Autodesk Inventor part; units mm, degrees
ref_plane "YZ Plane" through (0, 0, 0) normal (1, 0, 0) x (0, 1, 0)
ref_plane "XZ Plane" through (0, 0, 0) normal (0, 1, 0) x (-1, 0, 0)
ref_plane "XY Plane" through (0, 0, 0) normal (0, 0, 1) x (1, 0, 0)
sketch "Sketch1" plane through (0, 0, 0) normal (0, 0, 1) x (1, 0, 0)
  line L0 (0, 0) -> (73.025, 0)
  line L1 (73.025, 0) -> (73.025, 25.4)
  line L2 (73.025, 25.4) -> (-25.4001, 76.2)
  line L3 (-25.4001, 76.2) -> (-45.7201, 60.9599)
  line L4 (-45.7201, 60.9599) -> (0, 0)
  circle A0 centre (60.325, 12.7) radius 3.3734
  circle A1 centre (34.925, 12.7) radius 3.3734
  circle A2 centre (2.54, 17.78) radius 3.3734
  circle A3 centre (-27.9401, 58.42) radius 3.3734
  line L5 (73.025, 12.7) -> (-9.525, 12.7) construction
  line L6 (-35.5601, 68.5799) -> (15.875, 0) construction
  line L7 (0, 0) -> (49.8292, 37.372) construction
  line L8 (20.32, 15.24) -> (12.7, 25.4) construction
  circle A4 centre (-12.7001, 38.1) radius 3.3734
  dimension "d0" = 73.025
  dimension "d1" = 25.4
  dimension "d2" = 25.4
  dimension "d3" = 76.2
  dimension "d4" = 126.87
  dimension "d5" = 6.7469
  dimension "d6" = 25.4
  dimension "d7" = 12.7
  dimension "d8" = 12.7
  dimension "d12" = 12.7
  dimension "d13" = 25.4
  dimension "d14" = 12.7
  dimension "d15" = 38.1
extrude "Extrusion1" add sketch "Sketch1" along normal blind 3.175 contours L4 L3 L2 L1 L0 | A4
properties part number "angle gusset plate"
Can you work these out from the model? Positions are in its coordinate system, mm. Give positions to 0.01 mm unless a question says otherwise; leave off trailing zeros. Order: outer loops, then holes, each group sorted by start corner. A loop starts at its lowest first (then second) coordinate and runs counter-clockwise, first axis right, second up. Notation, with made-up numbers: (83, -31) - (97, -31) arc R29 cw to (97, 2) - close; hole circle Ø2 at (57.25, 76). An arc over 180 degrees is marked (long way). Use a Markdown table: item, result. Add a question column.
Q1. Please list where these lines run through material, in increasing order: line 1 along X through (y, z) = (14, 2.5) (3 decimals); line 2 along Y through (x, z) = (2.54, 1.05); line 3 along Y through (x, z) = (36, 1.85).
Q2. If we section it at B-B on y = 17.78: Write out the boundary of the cut face in (x, z) (3 decimals), plus the area to 3 significant figures.
Q3. If we section it at A-A on z = 0.55: Write out the boundary of the cut face in (x, y) (3 decimals).
Q4. If we section it at D-D on y = 39.5: Write out the boundary of the cut face in (x, z) (3 decimals), plus the area to 3 significant figures.
Q5. I'm going to push flat-ended pins straight in: pin 1 (4 mm diameter, centred on x = -27.94, y = 58.42, fed in from +Z); pin 2 (11 mm diameter, centred on x = 60.325, y = 12.7, fed in from +Z) (3 decimals). Where does each tip first touch, or does it pass through?
Q6. If we mould it in two halves opening along X, with no side actions, what happens to faces 1 (the flat face through (-23.18, 30.907, 1.565)), 2 (the cylindrical face through (34.194, 15.993, 1.565)), 3 (the flat face through (36, 0, 2))? For each: released by +X, released by -X, zero draft, split by the parting line, or undercut.
Q7. If we section it at C-C on x = 2.54: Write out the boundary of the cut face in (y, z) (3 decimals), plus the area to 3 significant figures.
Answers follow:
| question | item | result |
|---|---|---|
| 1 | line 1 | x = -10.5 to 31.812, 38.038 to 57.212, 63.438 to 73.025 |
| 1 | line 2 | y = 0 to 14.41, 21.15 to 61.78 |
| 1 | line 3 | y = 0 to 9.5, 15.9 to 44.51 |
| 2 | outline | (-13.335, 0) - (-0.833, 0) - (-0.833, 3.175) - (-13.335, 3.175) - close; (5.913, 0) - (73.025, 0) - (73.025, 3.175) - (5.913, 3.175) - close |
| 2 | area | 253 mm^2 |
| 3 | outline | (-45.72, 60.96) - (0, 0) - (73.025, 0) - (73.025, 25.4) - (-25.4, 76.2) - close; hole circle Ø6.747 at (-27.94, 58.42); hole circle Ø6.747 at (2.54, 17.78); hole circle Ø6.747 at (34.925, 12.7); hole circle Ø6.747 at (60.325, 12.7) |
| 4 | outline | (-29.625, 0) - (45.706, 0) - (45.706, 3.175) - (-29.625, 3.175) - close |
| 4 | area | 239 mm^2 |
| 5 | pin 1 | passes through |
| 5 | pin 2 | stops at z = 3.175 |
| 6 | face 1 | released by -X |
| 6 | face 2 | undercut |
| 6 | face 3 | zero draft |
| 7 | outline | (0, 0) - (14.407, 0) - (14.407, 3.175) - (0, 3.175) - close; (21.153, 0) - (61.779, 0) - (61.779, 3.175) - (21.153, 3.175) - close |
| 7 | area | 175 mm^2 |
